from build123d import *
from build123d.topology import SkipClean

# Parameters (mm, degrees)
BOSS_EXTRUDE1_DEPTH     = 3.81
SKETCH2_R               = 1.5875
BOSS_EXTRUDE2_DEPTH     = 4.7625
MIRROR2_COPY_1_SKETCH_R = 1.5875
MIRROR2_COPY_1_DEPTH    = 4.7625


with BuildPart() as part:
    # Sketch1 → Boss-Extrude1 (new body, symmetric)
    with BuildSketch(Plane.XY):
        with BuildLine():
            Line((9.65327, 1.5875), (-9.65327, 1.5875))
            ThreePointArc((-9.65327, 1.5875), (-11.24077, 0), (-9.65327, -1.5875))
            Line((-9.65327, -1.5875), (9.65327, -1.5875))
            ThreePointArc((9.65327, -1.5875), (11.24077, 0), (9.65327, 1.5875))
        make_face()
    extrude(amount=BOSS_EXTRUDE1_DEPTH, both=True)

    # Sketch2 → Boss-Extrude2 (add)
    with SkipClean():  # keep this step's faces unmerged: merging them makes the solid invalid here
        with BuildSketch(Plane.XY.offset(3.81)):
            with Locations(Location((-9.65327, 0, 0), (0, 0, 270))):  # turned: the seam where the file's is
                Circle(SKETCH2_R)
        boss_extrude2 = extrude(amount=BOSS_EXTRUDE2_DEPTH)

    # Mirror1: Boss-Extrude2 across plane
    with SkipClean():  # keep this step's faces unmerged: merging them makes the solid invalid here
        add(boss_extrude2.mirror(Plane(origin=(0, 0, 0), x_dir=(0, 0, 1), z_dir=(1, 0, 0))))

    # Mirror2: Boss-Extrude2 across plane
    with SkipClean():  # keep this step's faces unmerged: merging them makes the solid invalid here
        add(boss_extrude2.mirror(Plane.XY))

    # Mirror2 copy 1 sketch → Mirror2 copy 1 (add)
    with SkipClean():  # keep this step's faces unmerged: merging them makes the solid invalid here
        with BuildSketch(Plane(origin=(0, 0, -3.81), x_dir=(-1, 0, 0), z_dir=(0, 0, -1))):
            with Locations(Location((-9.65327, 0, 0), (0, 0, 270))):  # turned: the seam where the file's is
                Circle(MIRROR2_COPY_1_SKETCH_R)
        extrude(amount=MIRROR2_COPY_1_DEPTH)


solid = part.part
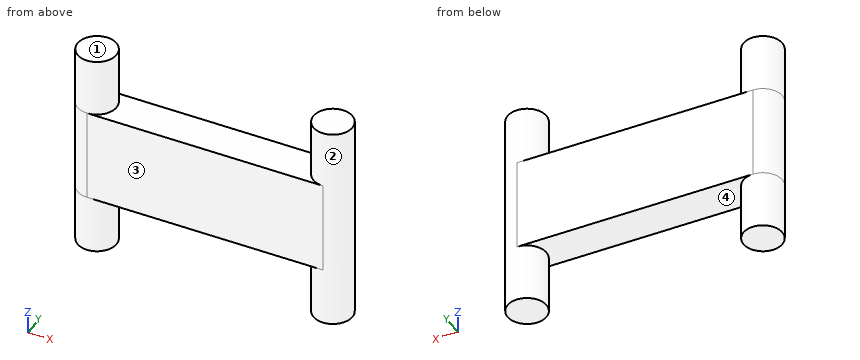
Model file for the job. Use its own axes, mm. Face numbers are marked on the shaded views. A direction names the side the tool comes from. Give positions to 0.01 mm unless a question says otherwise; leave off trailing zeros. Loops run counter-clockwise (first coordinate to the right, second up) from the corner with the lowest first, then second, coordinate; pieces in that order, holes last. Notation, with made-up numbers: (3.5, 0.25) -> (56.5, 0.25) arc R12 cw to (56.5, 17.25) -> close; hole circle Ø1 at (-20.5, 1.5). An arc over 180 degrees is marked (long way). Use a Markdown table: item, result. Add a question column.
(1) Drop flat-ended pins along their axis: pin 1 Ø1 at (x, y) = (-0.5, 0) entering from +Z; pin 2 Ø1 at (y, z) = (1, 5.5) entering from +X. Give the stop position or say it passes through.
(2) Wall check: line 1 along Z through (x, y) = (6, -0.5); line 2 along X through (y, z) = (0.7, 4); line 3 along X through (y, z) = (-1.1, -7.25). Give the ranges that are in metal, low to high.
(3) Slice it at C-C on x = -8.75. List the corners of the cut face in (y, z).
(4) Slice it at A-A on y = 0. List the corners of the cut face in (x, z), and give its area (3 significant figures).
(5) Slice it at D-D on z = 2. List the corners of the cut face in (x, y) (1 decimal).
(6) Slice it at B-B on z = -4.75. List the corners of the cut face in (x, y) (1 decimal), and give its area (3 significant figures).
(7) Tool access for the marked faces 1 and 2: list every direction of +Z, -Z, +X, -X, +Y, -Y with a clear straight run to the whole face (end or side of a thin tool).
(8) Mould opens along X. For the marked faces 3 and 4 say: +X half, -X half, draft (parallel to the pull), parting line (faces both ways), or undercut.
Filled sheet:
| question | item | result |
|---|---|---|
| 1 | pin 1 | z = 3.81 |
| 1 | pin 2 | x = 11.16 |
| 2 | line 1 | -3.81 to 3.81 |
| 2 | line 2 | -11.08 to -8.23, 8.23 to 11.08 |
| 2 | line 3 | -10.8 to -8.51, 8.51 to 10.8 |
| 3 | outline | (-1.59, -3.81) -> (-1.31, -3.81) -> (-1.31, -8.57) -> (1.31, -8.57) -> (1.31, -3.81) -> (1.59, -3.81) -> (1.59, 3.81) -> (1.31, 3.81) -> (1.31, 8.57) -> (-1.31, 8.57) -> (-1.31, 3.81) -> (-1.59, 3.81) -> close |
| 4 | outline | (-11.24, -8.57) -> (-8.07, -8.57) -> (-8.07, -3.81) -> (8.07, -3.81) -> (8.07, -8.57) -> (11.24, -8.57) -> (11.24, 8.57) -> (8.07, 8.57) -> (8.07, 3.81) -> (-8.07, 3.81) -> (-8.07, 8.57) -> (-11.24, 8.57) -> close |
| 4 | area | 232 mm2 |
| 5 | outline | (-9.7, -1.6) -> (9.7, -1.6) arc R1.6 ccw to (9.7, 1.6) -> (-9.7, 1.6) arc R1.6 ccw to start |
| 6 | outline | circle Ø3.2 at (-9.7, 0); circle Ø3.2 at (9.7, 0) |
| 6 | area | 15.8 mm2 |
| 7 | face 1 | +Z, +X, -X, +Y, -Y |
| 7 | face 2 | none |
| 8 | face 3 | draft |
| 8 | face 4 | undercut |
